from build123d import *

# Parameters (mm, degrees)
BOSS_EXTRUDE1_DEPTH = 1.5


with BuildPart() as part:
    # Sketch2 → Boss-Extrude1 (new, symmetric)
    with BuildSketch(Plane.XY):
        with BuildLine():
            Line((299.5, -67.353443934), (293.5, -67.353443934))
            ThreePointArc((293.5, -67.353443934), (292.085786438, -67.939230372), (291.5, -69.353443934))
            Line((291.5, -69.353443934), (291.5, -85.649534053))
            Line((291.5, -85.649534053), (281.5, -85.649534053))
            Line((281.5, -85.649534053), (281.5, -70.504592149))
            ThreePointArc((281.5, -70.504592149), (280.757064897, -67.882112699), (278.749040614, -66.038966065))
            ThreePointArc((278.749040614, -66.038966065), (170.034876315, -25.766389615), (55.097618142, -10.598112953))
            ThreePointArc((55.097618142, -10.598112953), (55.000467449, -10.596696958), (54.903307584, -10.596224945))
            Line((54.903307584, -10.596224945), (25, -10.596224945))
            Line((25, -10.596224945), (25, -3.5))
            Line((25, -3.5), (45, -3.5))
            Line((45, -3.5), (45, -0.5))
            ThreePointArc((45, -0.5), (176.353256324, -17.04581533), (299.5, -65.649534053))
            Line((299.5, -65.649534053), (299.5, -67.353443934))
        make_face()
    extrude(amount=BOSS_EXTRUDE1_DEPTH, both=True)


solid = part.part
The model under review builds one solid part; all positions refer to its coordinate system, in mm. Round coordinates to 2 decimals unless told otherwise and drop trailing zeros. Loops run counter-clockwise (first coordinate to the right, second up) from the corner with the lowest first, then second, coordinate; pieces in that order, holes last. Notation, with made-up numbers: (-30, 42.25) -> (10, 42.25) arc R24 ccw to (10, 67.25) -> close; hole circle Ø3 at (-30.75, 58). An arc over 180 degrees is marked (long way). One line per question, with ' | ' between items. Start each with the question number.
Item 1: Add section B-B, the plane x = 237. Write out the cut boundary in (y, z).
Item 2: Add section A-A, the plane z = 0.55. Write out the cut boundary in (x, y).
Item 3: Wall thickness on line 1 along X through (y, z) = (-70, 0.95); line 2 along Y through (x, z) = (78.5, -1.3); line 3 along Y through (x, z) = (285.5, -0.55): over which ranges is each line inside the solid? List them lowest first. Write a range as [from, to].
Item 4: Add section C-C, the plane y = -26.5. Write out the cut boundary in (x, z), then the cut area to 3 significant figures.
Item 5: For pin 1 (0.9 mm diameter, centred on y = -79, z = 0, fed in from -X); pin 2 (1.5 mm diameter, centred on y = -2, z = 0, fed in from -X), all flat-tipped, find the tip position at first contact; note any pin that passes through.
Return value:
1) outline: (-47.27, -1.5) -> (-36.52, -1.5) -> (-36.52, 1.5) -> (-47.27, 1.5) -> close
2) outline: (25, -10.6) -> (54.9, -10.6) arc R10 cw to (55.1, -10.6) arc R519.66 cw to (278.75, -66.04) arc R5 cw to (281.5, -70.5) -> (281.5, -85.65) -> (291.5, -85.65) -> (291.5, -69.35) arc R2 cw to (293.5, -67.35) -> (299.5, -67.35) -> (299.5, -65.65) arc R529.66 ccw to (45, -0.5) -> (45, -3.5) -> (25, -3.5) -> close
3) line 1: x = [281.47, 291.5] | line 2: y = [-11.58, -1.56] | line 3: y = [-85.65, -58.25]
4) outline: (172.96, -1.5) -> (208.91, -1.5) -> (208.91, 1.5) -> (172.96, 1.5) -> close | area: 108 mm2
5) pin 1: stops at x = 281.5 | pin 2: stops at x = 45
